Geometry check sheet. Reference: the model listing, model coordinates, mm. Face numbers are marked on the shaded views. Round coordinates to 2 decimals unless told otherwise and drop trailing zeros. Write each loop counter-clockwise with the first axis right and the second up, starting at its lowest first coordinate (ties: lowest second). Pieces come first, ordered by that corner, then holes.
Item 1: Cross-section at B-B (z = 22.25). Enter the section's corners in (x, y).
Item 2: Scan lines: probe 1 along Y at (x, z) = (-29, 8.75); probe 2 along X at (y, z) = (-1.5, 17); probe 3 along X at (y, z) = (-8, 2). Record each from-to range of solid material in increasing order.
Item 3: Depth check by flat-ended pin: P1, Ø6.5, axis at y = 0, z = 7.5, coming from the +X side; P2, Ø1.1, axis at x = 14.5, z = 11, coming from the +Y side; P3, Ø0.5, axis at x = 15, z = 14.5, coming from the -Y side. Enter the tip coordinate at first touch or a pass-through.
Item 4: Cross-section at A-A (x = -29). Enter the section's corners in (y, z), then the cut area to 4 significant figures.
Item 5: Draft check along Y on the marked faces 1, 2 and 3. Enter one of: pulls with the +Y half, pulls with the -Y half, needs draft (parallel to the pull), parting line crosses it, or undercut.
Item 6: Cross-section at C-C (y = 0). Enter the section's corners in (x, z), then the cut area to 3 significant figures.
Item 7: Cross-section at D-D (z = 7.5). Enter the section's corners in (x, y).
from build123d import *

# Parameters (mm, degrees)
ESQUISSE1_R             = 2
BOSS_EXTRU_1_DEPTH      = 25
ESQUISSE5_R             = 2
ENL_V_MAT_EXTRU_2_DEPTH = 10
CONG_1_R                = 5
CONG_2_R                = 1


with BuildPart() as part:
    # Esquisse1 → Boss.-Extru.1 (new body)
    with BuildSketch(Plane.XY):
        with BuildLine():
            Line((13.4187369, 3), (16.479153498, 3))
            ThreePointArc((16.479153498, 3), (10.731088016, 12.861036117), (0, 16.75))
            Line((0, 16.75), (-43.75, 16.75))
            Line((-43.75, 16.75), (-43.75, -16.75))
            Line((-43.75, -16.75), (0, -16.75))
            ThreePointArc((0, -16.75), (10.731088016, -12.861036117), (16.479153498, -3))
            Line((16.479153498, -3), (13.4187369, -3))
            ThreePointArc((13.4187369, -3), (-13.75, 0), (13.4187369, 3))
        make_face()
        with Locations((-29, 0)):
            Circle(ESQUISSE1_R, mode=Mode.SUBTRACT)
        with Locations((-19, 0)):
            Circle(ESQUISSE1_R, mode=Mode.SUBTRACT)
    extrude(amount=BOSS_EXTRU_1_DEPTH)

    # Esquisse5 → Enlèv. mat.-Extru.2 (cut)
    with BuildSketch(Plane.ZY.offset(43.75)):
        with Locations((7.5, 0)):
            Circle(ESQUISSE5_R)
        with Locations((17.5, 0)):
            Circle(ESQUISSE5_R)
    extrude(amount=-ENL_V_MAT_EXTRU_2_DEPTH, mode=Mode.SUBTRACT)

    # Congé1
    cong_1_edges = [part.edges().sort_by_distance(p)[0] for p in [
        (-43.75, -16.75, 12.5),
        (-43.75, 16.75, 12.5),
    ]]
    fillet(cong_1_edges, radius=CONG_1_R)

    # Congé2
    cong_2_edges = [part.edges().sort_by_distance(p)[0] for p in [
        (13.4187369, -3, 12.5),
        (16.479153498, -3, 12.5),
        (16.479153498, 3, 12.5),
        (13.4187369, 3, 12.5),
    ]]
    fillet(cong_2_edges, radius=CONG_2_R)


solid = part.part
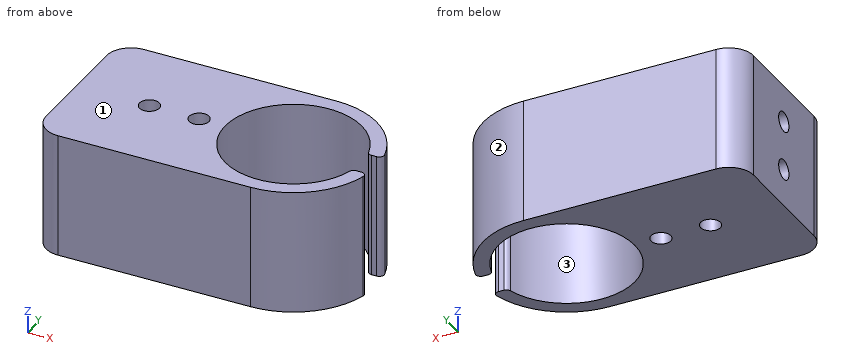
Resolved:
1. outline: (-43.75, -11.75) arc R5 ccw to (-38.75, -16.75) - (0, -16.75) arc R16.75 ccw to (16.2, -4.25) arc R1 ccw to (15.23, -3) - (14.2, -3) arc R1 ccw to (13.23, -3.73) arc R13.75 cw (long way) to (13.23, 3.73) arc R1 ccw to (14.2, 3) - (15.23, 3) arc R1 ccw to (16.2, 4.25) arc R16.75 ccw to (0, 16.75) - (-38.75, 16.75) arc R5 ccw to (-43.75, 11.75) - close; hole circle Ø4 at (-29, 0); hole circle Ø4 at (-19, 0)
2. probe 1: y = -16.75 to -2, 2 to 16.75
2. probe 2: x = -33.75 to -30.32, -27.68 to -20.32, -17.68 to -13.67
2. probe 3: x = -43.75 to -11.18, 11.18 to 14.72
3. P1: stops at x = 15.9
3. P2: stops at y = 9.27
3. P3: stops at y = -7.94
4. outline: (-16.75, 0) - (-2, 0) - (-2, 25) - (-16.75, 25) - close; (2, 0) - (16.75, 0) - (16.75, 25) - (2, 25) - close
4. area: 737.5 mm2
5. face 1: needs draft
5. face 2: pulls with the +Y half
5. face 3: undercut
6. outline: (-43.75, 0) - (-31, 0) - (-31, 25) - (-43.75, 25) - (-43.75, 19.5) - (-33.75, 19.5) - (-33.75, 15.5) - (-43.75, 15.5) - (-43.75, 9.5) - (-33.75, 9.5) - (-33.75, 5.5) - (-43.75, 5.5) - close; (-27, 0) - (-21, 0) - (-21, 25) - (-27, 25) - close; (-17, 0) - (-13.75, 0) - (-13.75, 25) - (-17, 25) - close
6. area: 470 mm2
7. outline: (-43.75, -11.75) arc R5 ccw to (-38.75, -16.75) - (0, -16.75) arc R16.75 ccw to (16.2, -4.25) arc R1 ccw to (15.23, -3) - (14.2, -3) arc R1 ccw to (13.23, -3.73) arc R13.75 cw (long way) to (13.23, 3.73) arc R1 ccw to (14.2, 3) - (15.23, 3) arc R1 ccw to (16.2, 4.25) arc R16.75 ccw to (0, 16.75) - (-38.75, 16.75) arc R5 ccw to (-43.75, 11.75) - (-43.75, 2) - (-33.75, 2) - (-33.75, -2) - (-43.75, -2) - close; hole circle Ø4 at (-29, 0); hole circle Ø4 at (-19, 0)
